from build123d import *

# Parameters (mm, degrees)
SALIENTE_EXTRUIR1_DEPTH = 3
CROQUIS2_R              = 1.125
CORTAR_EXTRUIR1_DEPTH   = 3


with BuildPart() as part:
    # Croquis1 → Saliente-Extruir1 (new body)
    with BuildSketch(Plane.XY):
        with BuildLine():
            Line((-6.25, 11.3), (6.25, 11.3))
            Line((6.25, 11.3), (6.25, 15.3))
            ThreePointArc((6.25, 15.3), (0.056504012, 17.109442987), (-5.670411261, 20.081970181))
            ThreePointArc((-5.670411261, 20.081970181), (-9.727780496, 20.258869159), (-11.848630151, 16.795412057))
            ThreePointArc((-11.848630151, 16.795412057), (-10.192303885, -28.221209783), (-3.713791608, -72.8))
            ThreePointArc((-3.713791608, -72.8), (-0.923786204, -75.3), (1.8662192, -72.8))
            ThreePointArc((1.8662192, -72.8), (4.506721754, -46.566008889), (7.954822861, -20.425902882))
            Line((7.954822861, -20.425902882), (6.25, -11.3))
            Line((6.25, -11.3), (-6.25, -11.3))
            Line((-6.25, -11.3), (-6.25, 11.3))
        make_face()
    extrude(amount=SALIENTE_EXTRUIR1_DEPTH)

    # Croquis2 → Cortar-Extruir1 (cut)
    with BuildSketch(Plane.XY.offset(3)):
        with Locations((0, 13.65)):
            Circle(CROQUIS2_R)
        with Locations((0, -13.65)):
            Circle(CROQUIS2_R)
    extrude(amount=-CORTAR_EXTRUIR1_DEPTH, mode=Mode.SUBTRACT)


solid = part.part
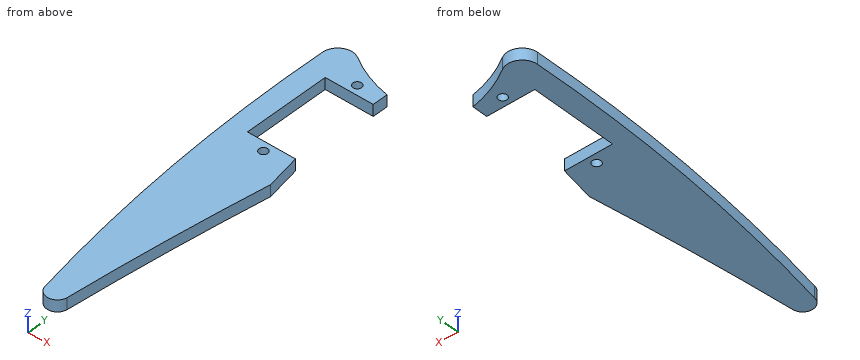
Build history of the part. All positions in model axes, mm. Coordinates: 2 decimals unless noted, no trailing zeros. Order: outer loops, then holes, each group sorted by start corner. A loop starts at its lowest first (then second) coordinate and runs counter-clockwise, first axis right, second up. Notation, with made-up numbers: M -30.75,-17 L 20.25,-17 A23 ccw 20.25,5 Z; hole C 77,81 d4. An arc over 180 degrees is marked long. One line per question, with ' | ' between items. Start each with the question number.
Q1. Probe L1, parallel to Y at x = 0, z = 1.35 (3 decimals); L2, parallel to Y at x = -2, z = 0.35; L3, parallel to Y at x = -2.75, z = 2.3. List the from-to ranges inside material, lowest first. Write a range as from..to.
Q2. Saw through at D-D (y = -13.65). List the corners of the cut face in (x, z) (3 decimals), then the cut area to 3 significant figures.
Q3. Saw through at B-B (x = 0). List the corners of the cut face in (y, z) (3 decimals).
Q4. Saw through at A-A (z = 2.4). Count the separate pieces of the cut face and the enclosed holes in it, then the cut area to 3 significant figures.
Q5. Saw through at C-C (y = 13.65). List the corners of the cut face in (x, z) (3 decimals), then the cut area to 3 significant figures.
Q6. Flat gauge pins, fed straight in: pin 1 Ø1 at (y, z) = (10, 1.5) entering from +X; pin 2 Ø2 at (x, y) = (0, 13.65) entering from -Z; pin 3 Ø3.5 at (x, y) = (0, -13.65) entering from +Z; pin 4 Ø0.9 at (y, z) = (13, 2) entering from +X. Where does each tip first touch, or does it go through?
Check values:
1) L1: y = -75.144..-14.775, -12.525..-11.3, 11.3..12.525, 14.775..17.132 | L2: y = -75.09..-11.3, 11.3..18.02 | L3: y = -74.62..-11.3, 11.3..18.39
2) outline: M -11.26,0 L -1.125,0 L -1.125,3 L -11.26,3 Z; M 1.125,0 L 6.689,0 L 6.689,3 L 1.125,3 Z | area: 47.1 mm2
3) outline: M -75.144,0 L -14.775,0 L -14.775,3 L -75.144,3 Z; M -12.525,0 L -11.3,0 L -11.3,3 L -12.525,3 Z; M 11.3,0 L 12.525,0 L 12.525,3 L 11.3,3 Z; M 14.775,0 L 17.132,0 L 17.132,3 L 14.775,3 Z
4) separate pieces: 1 | enclosed holes: 2 | area: 1,070 mm2
5) outline: M -11.89,0 L -1.125,0 L -1.125,3 L -11.89,3 Z; M 1.125,0 L 6.25,0 L 6.25,3 L 1.125,3 Z | area: 47.7 mm2
6) pin 1: stops at x = -6.25 | pin 2: passes through | pin 3: stops at z = 3 | pin 4: stops at x = 6.25
